Can you work these out from the model? Positions are in its coordinate system, mm. A direction names the side the tool comes from. Coordinates: 2 decimals unless noted, no trailing zeros. Order: outer loops, then holes, each group sorted by start corner. A loop starts at its lowest first (then second) coordinate and runs counter-clockwise, first axis right, second up. Notation, with made-up numbers: M 64,52.25 L 85,52.25 A18 cw 85,71.25 Z; hole C -18,4.25 d6. An arc over 180 degrees is marked long. Answer as a JSON object with one key per item and string values.
Autodesk Inventor part; units mm, degrees
ref_plane "YZ Plane" through (0, 0, 0) normal (1, 0, 0) x (0, 1, 0)
ref_plane "XZ Plane" through (0, 0, 0) normal (0, 1, 0) x (-1, 0, 0)
ref_plane "XY Plane" through (0, 0, 0) normal (0, 0, 1) x (1, 0, 0)
sketch "Sketch1" plane through (0, 0, 0) normal (0, 1, 0) x (-1, 0, 0)
  circle A0 centre (0, 0) radius 18
  circle A1 centre (0, 0) radius 23
  line L0 (-98, 65) -> (-18, 65)
  line L1 (-18, 65) -> (-18, 0)
  line L2 (-98, 0) -> (-98, 65)
  line L3 (-23, 60) -> (-93, 60)
  line L4 (-93, 60) -> (-93, 0)
  line L5 (-23, 0) -> (-23, 60)
  line L6 (-93, 0) -> (-98, 0)
  line L7 (-18, 60) -> (-10.0531, 14.931)
  line L8 (23, 0) -> (-23, 0)
  point P0 (18, 0)
  point P1 (-10.9836, 20.2079)
  point P2 (-18, 14.3178)
  dimension "d0" = 36
  dimension "d1" = 5
  dimension "d10" = 5
  dimension "d11" = 5
  dimension "d13" = 60
  dimension "d14" = 70
  dimension "d15" = 10
extrude "Extrusion1" add sketch "Sketch1" along normal mid plane 25.4 contours L8 A1 A0 | A0 L1 A1 L7 | L8 A1 L1 | A1 L5 L3 L4 L6 L2 L0 L1
fillet "Fillet1" radius 7.0104 1 edges at (18, 0, 14.3178)
extrude "Extrusion2" add sketch "Sketch1" along normal mid plane 3 contours A1 L1 L7
chamfer "Chamfer1" distance 3 angle 45 4 edges at (15.9446, 1.5, 22.2591) (18, 1.5, 43.6092) (15.9446, -1.5, 22.2591) (18, -1.5, 43.6092)
fillet "Fillet2" radius 2.5 11 edges at (18, 0, 65) (98, 0, 65) (98, 0, 0) (93, 0, 0) (23, 0, 60) (93, 0, 60) (-18, 0, 0) (-23, 0, 0) (10.0531, 0, 14.931) (10.9836, 8.6, 20.2079) (10.9836, -8.6, 20.2079)
equation "\"d10\" = d1"
equation "\"d11\" = d1"
properties part number "Clip"
Item 1: Which directions (+Z, -Z, +X, -X, +Y, -Y) give clear straight access to the entire face, cutting with the end or side of a thin tool? Please do faces 1 (the cylindrical face through (16.43, 8.54, 22.8)), 2 (the cylindrical face through (93.752, 0.178, 0.713)), 3 (the flat face through (16.5, -3, 39.7)).
Answers follow:
{"face 1": "+Z, -X, +Y", "face 2": "-Z, +Y, -Y", "face 3": "+Z, -X, -Y"}
Item 2: I want a section at B-B, the plane z = 6. Write out the boundary of the cut face in (x, y), plus the area to 3 significant figures.
Answers follow:
{"outline": "M 16.97,-12.7 L 23,-12.7 L 23,12.7 L 16.97,12.7 Z; M 93,-12.7 L 98,-12.7 L 98,12.7 L 93,12.7 Z", "area": "280 mm^2"}
Item 3: I want a section at D-D, the plane z = 37. Write out the boundary of the cut face in (x, y).
Answers follow:
{"outline": "M 13.94,-1.5 L 15,-1.5 L 18,-4.5 L 18,-12.7 L 23,-12.7 L 23,12.7 L 18,12.7 L 18,4.5 L 15,1.5 L 13.94,1.5 Z; M 93,-12.7 L 98,-12.7 L 98,12.7 L 93,12.7 Z"}
Item 4: Please list where these lines run through material, in increasing order: line 1 (Z direction, x = 63, y = -4.25); line 2 (Z direction, x = -1, y = 1.75); line 3 (X direction, y = 3.25, z = -16).
Answers follow:
{"line 1": "z = 60 to 65", "line 2": "z = -22.98 to -17.97", "line 3": "x = -16.52 to -8.25, 8.25 to 16.52"}
Item 5: I want a section at C-C, the plane x = 0. Write out the boundary of the cut face in (y, z), plus the area to 3 significant figures.
Answers follow:
{"outline": "M -12.7,-23 L 12.7,-23 L 12.7,-18 L -12.7,-18 Z", "area": "127 mm^2"}
Item 6: If we mould it in two halves opening along X, with no side actions, what happens to faces 4 (the cylindrical face through (0.92, -0.18, -22.98)), 5 (the flat face through (14, 1.5, 31)), 6 (the cylindrical face through (92.248, 0.178, 59.287))? For each: pulls with the +X half, pulls with the -X half, needs draft (parallel to the pull), parting line crosses it, or undercut.
Answers follow:
{"face 4": "parting line crosses it", "face 5": "needs draft", "face 6": "undercut"}
Item 7: I'm going to push flat-ended pins straight in: pin 1 (7.5 mm diameter, centred on x = 54, y = 5, fed in from -Z); pin 2 (1.7 mm diameter, centred on x = 13, z = 30.5, fed in from +Y); pin 3 (3 mm diameter, centred on x = 12.5, z = 31, fed in from -Y); pin 4 (21.5 mm diameter, centred on x = 0, z = 0, fed in from +Y). Where does each tip first touch, or does it pass through?
Answers follow:
{"pin 1": "stops at z = 60", "pin 2": "stops at y = 1.5", "pin 3": "stops at y = -1.5", "pin 4": "passes through"}
